CAD build for the part. Positions are in the model's coordinates, mm. A direction names the side the tool comes from. Coordinates: 2 decimals unless noted, no trailing zeros. Write each loop counter-clockwise with the first axis right and the second up, starting at its lowest first coordinate (ties: lowest second). Pieces come first, ordered by that corner, then holes. Notation, with made-up numbers: (-36.5, 19) - (-18.5, 19) arc R19 cw to (-18.5, 54) - close; hole circle Ø8 at (16.25, 44.25). An arc over 180 degrees is marked (long way). One line per question, with ' | ' between items. Start each with the question number.
1. Band-saw the part on B-B, the plane x = 67.5. Write the cut outline in (y, z).
2. Which spindle directions (+Z, -Z, +X, -X, +Y, -Y) get a long thin tool onto all of the face, cutting with end or side? Do faces 1 (the flat face through (-29, 0, 0)), 2 (the flat face through (80, -5, 0)). Say none if no direction does.
3. Band-saw the part on A-A, the plane z = 0. Write the cut outline in (x, y), then the cut area to 3 significant figures.
4. Band-saw the part on C-C, the plane y = -6.75. Write the cut outline in (x, z).
5. Flat gauge pins, fed straight in: P1, Ø1, axis at x = -37.5, z = 5, coming from the -Y side; P2, Ø7.5, axis at x = 67.5, z = 0, coming from the +Y side. Where does each tip first touch, or does it go through?
6. Band-saw the part on D-D, the plane x = 12. Write the cut outline in (y, z), then the cut area to 3 significant figures.
7. Probe line 1 (Z direction, x = 67.5, y = -6.75); line 2 (Y direction, x = -71, z = -10.25); line 3 (X direction, y = 2.25, z = -3). List the from-to ranges inside material, lowest first.
from build123d import *
from build123d.topology import SkipClean

# Parameters (mm, degrees)
SKETCH1_W           = 160
SKETCH1_H           = 25
SKETCH1_R           = 6.25
BOSS_EXTRUDE1_DEPTH = 4
BOSS_EXTRUDE2_START = 13
SKETCH2_W           = 56.41
SKETCH2_H           = 25
SKETCH2_R           = 6.25
BOSS_EXTRUDE2_DEPTH = 13
CHAMFER1_SIZE       = 10
CHAMFER1_SIZE2      = 30.776835372
FILLET1_R           = 10


with BuildPart() as part:
    # Sketch1 → Boss-Extrude1 (new body)
    with BuildSketch(Plane(origin=(0, 0, 0), x_dir=(1, 0, 0), z_dir=(0, 1, 0))):
        Rectangle(SKETCH1_W, SKETCH1_H)
        with Locations(Location((67.5, 0, 0), (0, 0, 270))):
            Circle(SKETCH1_R, mode=Mode.SUBTRACT)
    extrude(amount=BOSS_EXTRUDE1_DEPTH)

    # Sketch2 → Boss-Extrude2 (add)
    with SkipClean():  # the faces are left unmerged after this step: merging them gives an invalid solid
        with BuildSketch(Plane.XZ.offset(BOSS_EXTRUDE2_START)):
            with Locations((51.795, 0)):
                Rectangle(SKETCH2_W, SKETCH2_H)
            with Locations((67.5, 0)):
                Circle(SKETCH2_R, mode=Mode.SUBTRACT)
        extrude(amount=-BOSS_EXTRUDE2_DEPTH)

    # Chamfer1
    chamfer1_edges = [part.edges().sort_by_distance(p)[0] for p in [
        (23.59, -13, 0),
    ]]
    chamfer1_side = [part.faces().sort_by_distance(p)[0] for p in [
        (23.59, -6.5, 0),
    ]]
    chamfer(chamfer1_edges, length=CHAMFER1_SIZE, length2=CHAMFER1_SIZE2, reference=chamfer1_side[0])

    # Fillet1
    # the kernel refuses this fillet: 10 mm, written as the material it takes off along each edge
    with BuildSketch(Plane(origin=(23.59, -3, 27.668583986), x_dir=(0.9510565162951544, -0.3090169943749446, 0), z_dir=(0, 0, -1))) as fillet1_piece_1:
        with BuildLine():
            CenterArc((6.067433594, -10), FILLET1_R, 90, 44.38277042)
            Line((-0.927050983, -2.853169549), (-1.066940675, -2.71023294))
            ThreePointArc((-1.066940675, -2.71023294), (-0.653736795, -1.364781376), (-0.190211303, 0.061803399))
            Line((-0.190211303, 0.061803399), (0, 0.2))
            Line((0, 0.2), (6.067433594, 0.2))
            Line((6.067433594, 0.2), (6.067433594, 0))
        make_face()
    extrude(amount=55.337167971, mode=Mode.SUBTRACT)


solid = part.part
Filled in:
1) outline: (-13, -12.5) - (4, -12.5) - (4, -6.25) - (-13, -6.25) - close; (-13, 6.25) - (4, 6.25) - (4, 12.5) - (-13, 12.5) - close
2) face 1: +Z, -Z, -X, -Y | face 2: +Z, -Z, +X, +Y, -Y
3) outline: (-80, 0) - (23.59, 0) arc R10 ccw to (29.36, -4.87) - (54.37, -13) - (61.25, -13) - (61.25, 4) - (-80, 4) - close; (73.75, -13) - (80, -13) - (80, 4) - (73.75, 4) - close | area: 1,000 mm²
4) outline: (35.13, -12.5) - (80, -12.5) - (80, 12.5) - (35.13, 12.5) - close; hole circle Ø12.5 at (67.5, 0)
5) P1: stops at y = 0 | P2: passes through
6) outline: (0, -12.5) - (4, -12.5) - (4, 12.5) - (0, 12.5) - close | area: 100 mm²
7) line 1: z = -12.5 to -6.25, 6.25 to 12.5 | line 2: y = 0 to 4 | line 3: x = -80 to 62.02, 72.98 to 80
